from build123d import *

# Parameters (mm, degrees)
F0_W     = 100
F0_H     = 100
F1_DEPTH = 50
F3_D     = 60
F4_R     = 9.99999


# Not quite as in the source:
# - a fillet or chamfer is up to 0.001 mm smaller than in the source, because OpenCascade refuses the exact size


with BuildPart() as f1:
    # F0 (on Front) → F1 (new body)
    with BuildSketch(Plane.XZ):
        with Locations((50, 50)):
            Rectangle(F0_W, F0_H)
    extrude(amount=F1_DEPTH)

    # F3 (through all)
    with Locations(Plane.XZ.offset(50)):
        with Locations((50, 50)):
            Hole(F3_D / 2)

    # F4 (radius 10 in the source; OpenCascade refuses exactly that, so slightly less here)
    f4_edges = [f1.edges().sort_by_distance(p)[0] for p in [
        (50, -50, 0),
        (0, -50, 50),
        (100, -50, 50),
        (50, -50, 100),
        (20, -50, 50),
        (50, 0, 0),
        (0, 0, 50),
        (100, 0, 50),
        (50, 0, 100),
        (20, 0, 50),
    ]]
    fillet(f4_edges, radius=F4_R)


solid = f1.part
The model under review builds one solid part; all positions refer to its coordinate system, in mm. Coordinates: 2 decimals unless noted, no trailing zeros. Order: outer loops, then holes, each group sorted by start corner. A loop starts at its lowest first (then second) coordinate and runs counter-clockwise, first axis right, second up. Notation, with made-up numbers: (-26.5, 57) -> (20.5, 57) arc R13 cw to (20.5, 73) -> close; hole circle Ø2 at (52.5, 36). An arc over 180 degrees is marked (long way). Answer in a Markdown table with one row per item.
(1) Consider section C-C (y = -38.5). Write out the cut boundary in (x, z), plus the area to 3 significant figures.
Answers:
| item | result |
|---|---|
| outline | (0, 0) -> (100, 0) -> (100, 100) -> (0, 100) -> close; hole circle Ø60 at (50, 50) |
| area | 7,170 mm² |
(2) Wall thickness on line 1 along Z through (x, y) = (50, -36); line 2 along Z through (x, y) = (72, -20); line 3 along X through (y, z) = (-39, 63): over which ranges is each line inside the solid? List them lowest first.
Answers:
| item | result |
|---|---|
| line 1 | 0 to 20, 80 to 100 |
| line 2 | 0 to 29.6, 70.4 to 100 |
| line 3 | 0 to 22.96, 77.04 to 100 |
(3) The part is to be moulded in two halves that separate along X. For faces 1 (the cylindrical face through (56.503, -24.79, 20.713)), 2 (the cylindrical face through (50.7, -46.99, 2.85)), 3 (the flat face through (0, -25, 49)), say which applies: +X half, -X half, draft (parallel to the pull), parting line (faces both ways), or undercut.
Answers:
| item | result |
|---|---|
| face 1 | undercut |
| face 2 | draft |
| face 3 | -X half |
(4) Insertion check: pin 1 (8 mm diameter, centred on x = 73, z = 29.5, fed in from -Y). The pin has a flat end and moves straight along its axis. Give the tip position at first contact, or say it passes through.
Answers:
| item | result |
|---|---|
| pin 1 | y = -48.55 |
(5) Consider section D-D (y = -45.5). Write out the cut boundary in (x, z).
Answers:
| item | result |
|---|---|
| outline | (1.65, 1.65) -> (98.35, 1.65) -> (98.35, 98.35) -> (1.65, 98.35) -> close; hole circle Ø63.3 at (50, 50) |
